from build123d import *

# Parameters (mm, degrees)
SKETCH_3_R      = 3
SKETCH_3_R_2    = 2
SKETCH_3_R_3    = 1.5
SKETCH_3_R_4    = 5
EXTRUDE_1_DEPTH = 2


with BuildPart() as part:
    # 草图3 → 凸台-拉伸1 (new body)
    with BuildSketch(Plane.XY):
        with BuildLine():
            Line((-45, -3.990216685), (-45, -19.82))
            Line((-45, -19.82), (-25, -39.82))
            Line((-25, -39.82), (-15, -39.82))
            ThreePointArc((-15, -39.82), (0, -54.82), (15, -39.82))
            Line((15, -39.82), (25, -39.82))
            Line((25, -39.82), (45, -19.82))
            Line((45, -19.82), (45, -3.990216685))
            Line((45, -3.990216685), (45, 31.317051182))
            Line((45, 31.317051182), (41, 39.152540881))
            Line((41, 39.152540881), (34.06116735, 39.152540881))
            ThreePointArc((34.06116735, 39.152540881), (-11.38853896, 19.746708007), (-37.576612526, 61.656694359))
            Line((-37.576612526, 61.656694359), (-46.5, 63))
            Line((-46.5, 63), (-46.5, 28.773494756))
            add(Edge.make_bspline(
                [(-45, 25.109783315), (-46.274240542, 26.725120767), (-46.5, 28.773494756)],
                knots=[0, 0, 0, 1, 1, 1], degree=2))
            Line((-45, 25.109783315), (-45, -3.990216685))
        make_face()
        with Locations((0, -1.82)):
            Circle(SKETCH_3_R, mode=Mode.SUBTRACT)
        with Locations((0, 13.5)):
            Circle(SKETCH_3_R_2, mode=Mode.SUBTRACT)
        with Locations((-30.0520382, 25.9479618)):
            Circle(SKETCH_3_R_2, mode=Mode.SUBTRACT)
        with Locations((-42.5, 56)):
            Circle(SKETCH_3_R_2, mode=Mode.SUBTRACT)
        with Locations((30.0520382, 25.9479618)):
            Circle(SKETCH_3_R_2, mode=Mode.SUBTRACT)
        with Locations((0, -20.82)):
            Circle(SKETCH_3_R, mode=Mode.SUBTRACT)
        with Locations((0, -39.82)):
            Circle(SKETCH_3_R, mode=Mode.SUBTRACT)
        with Locations((-25, -1.990216685)):
            Circle(SKETCH_3_R_3, mode=Mode.SUBTRACT)
        with Locations((-25, -19.82)):
            Circle(SKETCH_3_R_3, mode=Mode.SUBTRACT)
        with Locations((-25, 13.509783315)):
            Circle(SKETCH_3_R_3, mode=Mode.SUBTRACT)
        with Locations(Location((25, 13.509783315, 0), (0, 0, 180))):
            Circle(SKETCH_3_R_3, mode=Mode.SUBTRACT)
        with Locations(Location((25, -19.82, 0), (0, 0, 180))):
            Circle(SKETCH_3_R_3, mode=Mode.SUBTRACT)
        with Locations(Location((25, -1.990216685, 0), (0, 0, 180))):
            Circle(SKETCH_3_R_3, mode=Mode.SUBTRACT)
        with Locations((-12.5, -11.405108343)):
            Circle(SKETCH_3_R_4, mode=Mode.SUBTRACT)
        with Locations((-12.5, 5.844891657)):
            Circle(SKETCH_3_R_4, mode=Mode.SUBTRACT)
        with Locations(Location((12.5, 5.844891657, 0), (0, 0, 180))):
            Circle(SKETCH_3_R_4, mode=Mode.SUBTRACT)
        with Locations(Location((12.5, -11.405108343, 0), (0, 0, 180))):
            Circle(SKETCH_3_R_4, mode=Mode.SUBTRACT)
        with BuildLine():
            Line((-41.6, -1.990216685), (-39.4, -1.990216685))
            Line((-39.4, -1.990216685), (-39.4, -10.190216685))
            ThreePointArc((-39.4, -10.190216685), (-40.5, -10.645851604), (-41.6, -10.190216685))
            Line((-41.6, -10.190216685), (-41.6, -1.990216685))
        make_face(mode=Mode.SUBTRACT)
        with BuildLine():
            Line((41.6, -10.190216685), (41.6, -1.990216685))
            Line((41.6, -1.990216685), (39.4, -1.990216685))
            Line((39.4, -1.990216685), (39.4, -10.190216685))
            ThreePointArc((39.4, -10.190216685), (40.5, -10.645851604), (41.6, -10.190216685))
        make_face(mode=Mode.SUBTRACT)
        with BuildLine():
            Line((39.4, 25.109783315), (39.4, 16.909783315))
            Line((39.4, 16.909783315), (41.6, 16.909783315))
            Line((41.6, 16.909783315), (41.6, 25.109783315))
            ThreePointArc((41.6, 25.109783315), (40.5, 25.565418233), (39.4, 25.109783315))
        make_face(mode=Mode.SUBTRACT)
        with BuildLine():
            Line((-41.6, 25.109783315), (-41.6, 16.909783315))
            Line((-41.6, 16.909783315), (-39.4, 16.909783315))
            Line((-39.4, 16.909783315), (-39.4, 25.109783315))
            ThreePointArc((-39.4, 25.109783315), (-40.5, 25.565418233), (-41.6, 25.109783315))
        make_face(mode=Mode.SUBTRACT)
    extrude(amount=EXTRUDE_1_DEPTH)


solid = part.part
Source: CAD feature listing. Evaluate the final solid. Frame: model axes, mm. Coordinates: 2 decimals unless noted, no trailing zeros. Write each loop counter-clockwise with the first axis right and the second up, starting at its lowest first coordinate (ties: lowest second). Pieces come first, ordered by that corner, then holes. Notation, with made-up numbers: M 15.25,-11 L 70.25,-11 A27 cw 70.25,17 Z; hole C -34.5,29.5 d6. An arc over 180 degrees is marked long. Use a Markdown table: item, result.
1) First-contact query: pin 1 Ø1 at (x, z) = (-40, 1.5) entering from -Y; pin 2 Ø3.5 at (x, y) = (-30.05, 25.95) entering from -Z; pin 3 Ø1 at (x, z) = (-40.5, 1) entering from +Y. Flat tips, straight axial feed; report the tip coordinate or a pass-through.
Conclusion:
| item | result |
|---|---|
| pin 1 | stops at y = -25.32 |
| pin 2 | passes through |
| pin 3 | stops at y = 62.17 |
2) Section C-C, the plane x = 12.5. Output: boundary loops of the cut face in (y, z), then the cut area to 3 significant figures.
Conclusion:
| item | result |
|---|---|
| outline | M -48.11,0 L -16.41,0 L -16.41,2 L -48.11,2 Z; M -6.41,0 L 0.84,0 L 0.84,2 L -6.41,2 Z; M 10.84,0 L 20.11,0 L 20.11,2 L 10.84,2 Z |
| area | 96.5 mm^2 |
3) Ray query, L1, parallel to Y at x = 0, z = 1.55; L2, parallel to X at y = 10, z = 1.6; L3, parallel to Y at x = 8, z = 1.7. Return the intervals inside material, ascending.
Conclusion:
| item | result |
|---|---|
| L1 | y = -54.82 to -42.82, -36.82 to -23.82, -17.82 to -4.82, 1.18 to 11.5, 15.5 to 18 |
| L2 | x = -45 to -15.28, -9.72 to 9.72, 15.28 to 45 |
| L3 | y = -52.51 to -13.58, -9.23 to 3.67, 8.02 to 18.85 |
4) Section B-B, the plane x = 0. Output: boundary loops of the cut face in (y, z).
Conclusion:
| item | result |
|---|---|
| outline | M -54.82,0 L -42.82,0 L -42.82,2 L -54.82,2 Z; M -36.82,0 L -23.82,0 L -23.82,2 L -36.82,2 Z; M -17.82,0 L -4.82,0 L -4.82,2 L -17.82,2 Z; M 1.18,0 L 11.5,0 L 11.5,2 L 1.18,2 Z; M 15.5,0 L 18,0 L 18,2 L 15.5,2 Z |
5) Section D-D, the plane y = -13. Output: boundary loops of the cut face in (x, z), then the cut area to 3 significant figures.
Conclusion:
| item | result |
|---|---|
| outline | M -45,0 L -17.24,0 L -17.24,2 L -45,2 Z; M -7.76,0 L 7.76,0 L 7.76,2 L -7.76,2 Z; M 17.24,0 L 45,0 L 45,2 L 17.24,2 Z |
| area | 142 mm^2 |
6) Mould query, pull axis X, two halves, no side actions, for faces 1 (the flat face through (-35.14, -29.68, 0.99)), 2 (the cylindrical face through (1.61, -37.29, 0.99)), 3 (the flat face through (-1, -8, 0)). Classes: pulls with the +X half, pulls with the -X half, needs draft (parallel to the pull), parting line crosses it, or undercut.
Conclusion:
| item | result |
|---|---|
| face 1 | pulls with the -X half |
| face 2 | undercut |
| face 3 | needs draft |
7) Section A-A, the plane y = 56. Output: boundary loops of the cut face in (x, z), then the cut area to 3 significant figures.
Conclusion:
| item | result |
|---|---|
| outline | M -46.5,0 L -44.5,0 L -44.5,2 L -46.5,2 Z; M -40.5,0 L -38,0 L -38,2 L -40.5,2 Z |
| area | 9.00 mm^2 |
